from build123d import *

# Parameters (mm, degrees)
BOSS_EXTRUDE2_DEPTH = 10
SKETCH3_R           = 10
CUT_EXTRUDE1_DEPTH  = 2.2
SKETCH4_R           = 2.5
CUT_EXTRUDE2_DEPTH  = 26.137532403


with BuildPart() as part:
    # Sketch2 → Boss-Extrude2 (new body)
    with BuildSketch(Plane(origin=(0, 0, 0), x_dir=(1, 0, 0), z_dir=(0, 1, 0))):
        with BuildLine():
            Line((-0.625, 16.897566915), (0.625, 16.897566915))
            Line((0.625, 16.897566915), (1.75, 14.897566915))
            ThreePointArc((1.75, 14.897566915), (2.346516976, 14.815325109), (2.939252448, 14.709207832))
            Line((2.939252448, 14.709207832), (4.627225018, 16.263676746))
            Line((4.627225018, 16.263676746), (5.816045663, 15.877405503))
            Line((5.816045663, 15.877405503), (6.267950255, 13.627648352))
            ThreePointArc((6.267950255, 13.627648352), (6.809857496, 13.365097863), (7.340790388, 13.081009001))
            Line((7.340790388, 13.081009001), (9.426505011, 14.037784581))
            Line((9.426505011, 14.037784581), (10.437776254, 13.303053015))
            Line((10.437776254, 13.303053015), (10.172349868, 11.023760618))
            ThreePointArc((10.172349868, 11.023760618), (10.606601718, 10.606601718), (11.023760618, 10.172349868))
            Line((11.023760618, 10.172349868), (13.303053015, 10.437776254))
            Line((13.303053015, 10.437776254), (14.037784581, 9.426505011))
            Line((14.037784581, 9.426505011), (13.081009001, 7.340790388))
            ThreePointArc((13.081009001, 7.340790388), (13.365097863, 6.809857496), (13.627648352, 6.267950255))
            Line((13.627648352, 6.267950255), (15.877405503, 5.816045663))
            Line((15.877405503, 5.816045663), (16.263676746, 4.627225018))
            Line((16.263676746, 4.627225018), (14.709207832, 2.939252448))
            ThreePointArc((14.709207832, 2.939252448), (14.815325109, 2.346516976), (14.897566915, 1.75))
            Line((14.897566915, 1.75), (16.897566915, 0.625))
            Line((16.897566915, 0.625), (16.897566915, -0.625))
            Line((16.897566915, -0.625), (14.897566915, -1.75))
            ThreePointArc((14.897566915, -1.75), (14.815325109, -2.346516976), (14.709207832, -2.939252448))
            Line((14.709207832, -2.939252448), (16.263676746, -4.627225018))
            Line((16.263676746, -4.627225018), (15.877405503, -5.816045663))
            Line((15.877405503, -5.816045663), (13.627648352, -6.267950255))
            ThreePointArc((13.627648352, -6.267950255), (13.365097863, -6.809857496), (13.081009001, -7.340790388))
            Line((13.081009001, -7.340790388), (14.037784581, -9.426505011))
            Line((14.037784581, -9.426505011), (13.303053015, -10.437776254))
            Line((13.303053015, -10.437776254), (11.023760618, -10.172349868))
            ThreePointArc((11.023760618, -10.172349868), (10.606601718, -10.606601718), (10.172349868, -11.023760618))
            Line((10.172349868, -11.023760618), (10.437776254, -13.303053015))
            Line((10.437776254, -13.303053015), (9.426505011, -14.037784581))
            Line((9.426505011, -14.037784581), (7.340790388, -13.081009001))
            ThreePointArc((7.340790388, -13.081009001), (6.809857496, -13.365097863), (6.267950255, -13.627648352))
            Line((6.267950255, -13.627648352), (5.816045663, -15.877405503))
            Line((5.816045663, -15.877405503), (4.627225018, -16.263676746))
            Line((4.627225018, -16.263676746), (2.939252448, -14.709207832))
            ThreePointArc((2.939252448, -14.709207832), (2.346516976, -14.815325109), (1.75, -14.897566915))
            Line((1.75, -14.897566915), (0.625, -16.897566915))
            Line((0.625, -16.897566915), (-0.625, -16.897566915))
            Line((-0.625, -16.897566915), (-1.75, -14.897566915))
            ThreePointArc((-1.75, -14.897566915), (-2.346516976, -14.815325109), (-2.939252448, -14.709207832))
            Line((-2.939252448, -14.709207832), (-4.627225018, -16.263676746))
            Line((-4.627225018, -16.263676746), (-5.816045663, -15.877405503))
            Line((-5.816045663, -15.877405503), (-6.267950255, -13.627648352))
            ThreePointArc((-6.267950255, -13.627648352), (-6.809857496, -13.365097863), (-7.340790388, -13.081009001))
            Line((-7.340790388, -13.081009001), (-9.426505011, -14.037784581))
            Line((-9.426505011, -14.037784581), (-10.437776254, -13.303053015))
            Line((-10.437776254, -13.303053015), (-10.172349868, -11.023760618))
            ThreePointArc((-10.172349868, -11.023760618), (-10.606601718, -10.606601718), (-11.023760618, -10.172349868))
            Line((-11.023760618, -10.172349868), (-13.303053015, -10.437776254))
            Line((-13.303053015, -10.437776254), (-14.037784581, -9.426505011))
            Line((-14.037784581, -9.426505011), (-13.081009001, -7.340790388))
            ThreePointArc((-13.081009001, -7.340790388), (-13.365097863, -6.809857496), (-13.627648352, -6.267950255))
            Line((-13.627648352, -6.267950255), (-15.877405503, -5.816045663))
            Line((-15.877405503, -5.816045663), (-16.263676746, -4.627225018))
            Line((-16.263676746, -4.627225018), (-14.709207832, -2.939252448))
            ThreePointArc((-14.709207832, -2.939252448), (-14.815325109, -2.346516976), (-14.897566915, -1.75))
            Line((-14.897566915, -1.75), (-16.897566915, -0.625))
            Line((-16.897566915, -0.625), (-16.897566915, 0.625))
            Line((-16.897566915, 0.625), (-14.897566915, 1.75))
            ThreePointArc((-14.897566915, 1.75), (-14.815325109, 2.346516976), (-14.709207832, 2.939252448))
            Line((-14.709207832, 2.939252448), (-16.263676746, 4.627225018))
            Line((-16.263676746, 4.627225018), (-15.877405503, 5.816045663))
            Line((-15.877405503, 5.816045663), (-13.627648352, 6.267950255))
            ThreePointArc((-13.627648352, 6.267950255), (-13.365097863, 6.809857496), (-13.081009001, 7.340790388))
            Line((-13.081009001, 7.340790388), (-14.037784581, 9.426505011))
            Line((-14.037784581, 9.426505011), (-13.303053015, 10.437776254))
            Line((-13.303053015, 10.437776254), (-11.023760618, 10.172349868))
            ThreePointArc((-11.023760618, 10.172349868), (-10.606601718, 10.606601718), (-10.172349868, 11.023760618))
            Line((-10.172349868, 11.023760618), (-10.437776254, 13.303053015))
            Line((-10.437776254, 13.303053015), (-9.426505011, 14.037784581))
            Line((-9.426505011, 14.037784581), (-7.340790388, 13.081009001))
            ThreePointArc((-7.340790388, 13.081009001), (-6.809857496, 13.365097863), (-6.267950255, 13.627648352))
            Line((-6.267950255, 13.627648352), (-5.816045663, 15.877405503))
            Line((-5.816045663, 15.877405503), (-4.627225018, 16.263676746))
            Line((-4.627225018, 16.263676746), (-2.939252448, 14.709207832))
            ThreePointArc((-2.939252448, 14.709207832), (-2.346516976, 14.815325109), (-1.75, 14.897566915))
            Line((-1.75, 14.897566915), (-0.625, 16.897566915))
        make_face()
    extrude(amount=BOSS_EXTRUDE2_DEPTH)

    # Sketch3 → Cut-Extrude1 (cut)
    with BuildSketch(Plane.XZ):
        with Locations(Location((0, 0, 0), (0, 0, 270))):
            Circle(SKETCH3_R)
    extrude(amount=-CUT_EXTRUDE1_DEPTH, mode=Mode.SUBTRACT)

    # Sketch4 → Cut-Extrude2 (cut, through all)
    with BuildSketch(Plane.XZ.offset(-2.2)):
        with Locations(Location((0, 0, 0), (0, 0, 270))):
            Circle(SKETCH4_R)
    extrude(amount=-CUT_EXTRUDE2_DEPTH, mode=Mode.SUBTRACT)


solid = part.part
Can you work these out from the model? Positions are in its coordinate system, mm. A direction names the side the tool comes from. Coordinates: 2 decimals unless noted, no trailing zeros. Loops run counter-clockwise (first coordinate to the right, second up) from the corner with the lowest first, then second, coordinate; pieces in that order, holes last. Notation, with made-up numbers: (32.5, 81.25) - (61.5, 81.25) arc R17 cw to (61.5, 93.25) - close; hole circle Ø7 at (-23, -10.5). An arc over 180 degrees is marked (long way). Put each result on its own line as item: value. Start each with the question number.
Item 1: Suppose I cut it at A-A (x = 0). Please give me the cut outline in (y, z).
Item 2: If I drill on line 1 along X through (y, z) = (8, 0); line 2 along X through (y, z) = (5.75, -15); line 3 along X through (y, z) = (1.45, 0), over which ranges is the centre line in solid material (lowest first)?
Item 3: If we mould it in two halves opening along X, with no side actions, what happens to faces 1 (the face through (-15.5, 4.9, 3.8)), 2 (the face through (-6.04, 4.93, 14.77)), 3 (the face through (9.939, 4.93, 13.665))? For each: +X half, -X half, draft (parallel to the pull), parting line (faces both ways), or undercut.
Item 4: Suppose I cut it at C-C (x = -12). Please give me the cut outline in (y, z), and give its area (3 significant figures).
Item 5: Which directions (+Z, -Z, +X, -X, +Y, -Y) give clear straight access to the entire face, cutting with the end or side of a thin tool? Please do faces 4 (the face through (-12.179, 4.93, -10.307)), 5 (the face through (6.045, 4.93, 14.737)), 6 (the face through (14.814, 4.93, -2.355)).
Item 6: Suppose I cut it at B-B (z = 0). Please give me the cut outline in (x, y).
Item 7: For pin 1 (5 mm diameter, centred on y = 6.5, z = -1, fed in from +X); pin 2 (5 mm diameter, centred on y = 8.5, z = 6, fed in from +X); pin 3 (3 mm diameter, centred on x = 0, z = 0, fed in from -Y); pin 4 (3 mm diameter, centred on x = 10, y = 3.5, fed in from +Z), each with a flat end and sliding along its axis, tell me the tip position at first contact or that it passes through.
Here are the results:
1. outline: (0, -16.9) - (10, -16.9) - (10, -2.5) - (2.2, -2.5) - (2.2, -10) - (0, -10) - close; (0, 10) - (2.2, 10) - (2.2, 2.5) - (10, 2.5) - (10, 16.9) - (0, 16.9) - close
2. line 1: -16.9 to -2.5, 2.5 to 16.9
2. line 2: -5.99 to -3.26, -1.69 to 1.69, 3.26 to 5.99
2. line 3: -16.9 to -10, 10 to 16.9
3. face 1: -X half
3. face 2: undercut
3. face 3: +X half
4. outline: (0, -10.29) - (10, -10.29) - (10, 10.29) - (0, 10.29) - close
4. area: 206 mm²
5. face 4: -Z, +Y, -Y
5. face 5: +Z, +Y, -Y
5. face 6: +X, +Y, -Y
6. outline: (-16.9, 0) - (-10, 0) - (-10, 2.2) - (-2.5, 2.2) - (-2.5, 10) - (-16.9, 10) - close; (2.5, 2.2) - (10, 2.2) - (10, 0) - (16.9, 0) - (16.9, 10) - (2.5, 10) - close
7. pin 1: x = 16.9
7. pin 2: x = 16.26
7. pin 3: through
7. pin 4: z = 14.04
